Geometry check sheet. Reference: the model listing, model coordinates, mm. Round coordinates to 2 decimals unless told otherwise and drop trailing zeros. One line per question, with ' | ' between items.
```python
from build123d import *

# Parameters (mm, degrees)
LOFT_START          = -150
LOFT_18_DEPTH       = 150
FILLET_1_R          = 50
SKETCH_8_W          = 150
SKETCH_8_H          = 89.90044461
CUT_EXTRUDE_3_DEPTH = 194.637322649
FILLET_3_R          = 10
EXTRUDE_1_REACH     = 195.637
SKETCH_5_R          = 5


# Read off the part's stored shape, not the designer's step: 放样18
with BuildPart() as part:
    # 放样18 outline → 放样18 (new body)
    with BuildSketch(Plane.YZ.offset(LOFT_START)):
        with BuildLine():
            Line((-92.019059125, 77.475043518), (-94.7292742, 73.273289807))
            add(Edge.make_bspline(
                [(-2.5, 0), (-30.482362978, 27.663701514), (-61.402130233, 52.230749004), (-94.7292742, 73.273289807)],
                knots=[0, 0, 0, 0, 1, 1, 1, 1], degree=3))
            Line((-2.5, 0), (2.5, 0))
            add(Edge.make_bspline(
                [(2.5, 0), (-26.24562462, 29.064286084), (-57.928653516, 55.031918144), (-92.019059125, 77.475043518)],
                knots=[0, 0, 0, 0, 1, 1, 1, 1], degree=3))
        make_face()
    extrude(amount=LOFT_18_DEPTH)

    # 圆角1
    fillet_1_edges = [part.edges().sort_by_distance(p)[0] for p in [
        (-150, -93.374166663, 75.374166663),
    ]]
    fillet(fillet_1_edges, radius=FILLET_1_R)

    # 草图8 → 切除-拉伸3 (cut, through all)
    with BuildSketch(Plane(origin=(0, -17.799060008, -17.799060008), x_dir=(-1, 0, 0), z_dir=(0, 0.7071067811865488, 0.7071067811865464))):
        with Locations((75, -43.182455352)):
            Rectangle(SKETCH_8_W, SKETCH_8_H)
    extrude(amount=CUT_EXTRUDE_3_DEPTH, mode=Mode.SUBTRACT)

    # 圆角3
    fillet_3_edges = [part.edges().sort_by_distance(p)[0] for p in [
        (0, -93.374166663, 75.374166663),
        (0, -1.246870677, 1.253129323),
        (-150, -1.246870677, 1.253129323),
    ]]
    fillet(fillet_3_edges, radius=FILLET_3_R)

    # 草图5 → 凸台-拉伸1 (add, up to next)
    with BuildSketch(Plane(origin=(0, -17.799060008, -17.799060008), x_dir=(-1, 0, 0), z_dir=(0, 0.7071067811865488, 0.7071067811865464)), mode=Mode.PRIVATE) as extrude_1_sk1:
        with Locations(Location((140, 11.767766953, 0), (0, 0, 270))):
            Circle(SKETCH_5_R)
    extrude_1_tool1 = extrude(extrude_1_sk1.sketch, amount=EXTRUDE_1_REACH, mode=Mode.PRIVATE) - part.part
    # 草图5 → 凸台-拉伸1 (add, up to next)
    with BuildSketch(Plane(origin=(0, -17.799060008, -17.799060008), x_dir=(-1, 0, 0), z_dir=(0, 0.7071067811865488, 0.7071067811865464)), mode=Mode.PRIVATE) as extrude_1_sk2:
        with Locations(Location((10, 11.767766953, 0), (0, 0, 270))):
            Circle(SKETCH_5_R)
    extrude_1_tool2 = extrude(extrude_1_sk2.sketch, amount=EXTRUDE_1_REACH, mode=Mode.PRIVATE) - part.part
    # 草图5 → 凸台-拉伸1 (add, up to next)
    with BuildSketch(Plane(origin=(0, -17.799060008, -17.799060008), x_dir=(-1, 0, 0), z_dir=(0, 0.7071067811865488, 0.7071067811865464)), mode=Mode.PRIVATE) as extrude_1_sk3:
        with Locations(Location((10, 110.037688609, 0), (0, 0, 270))):
            Circle(SKETCH_5_R)
    extrude_1_tool3 = extrude(extrude_1_sk3.sketch, amount=EXTRUDE_1_REACH, mode=Mode.PRIVATE) - part.part
    # 草图5 → 凸台-拉伸1 (add, up to next)
    with BuildSketch(Plane(origin=(0, -17.799060008, -17.799060008), x_dir=(-1, 0, 0), z_dir=(0, 0.7071067811865488, 0.7071067811865464)), mode=Mode.PRIVATE) as extrude_1_sk4:
        with Locations(Location((100, 70.425532461, 0), (0, 0, 270))):
            Circle(SKETCH_5_R)
    extrude_1_tool4 = extrude(extrude_1_sk4.sketch, amount=EXTRUDE_1_REACH, mode=Mode.PRIVATE) - part.part
    add(extrude_1_tool1.solids().sort_by_distance((-140, -26.120128, -9.477992))[0])
    add(extrude_1_tool2.solids().sort_by_distance((-10, -26.120128, -9.477992))[0])
    add(extrude_1_tool3.solids().sort_by_distance((-10, -95.607456, 60.009336))[0])
    add(extrude_1_tool4.solids().sort_by_distance((-100, -67.597432, 31.999312))[0])


solid = part.part
```
(1) Sectioned sample at A-A on y = -14.5. Count the separate pieces of the cut face and the enclosed holes in it, then the cut area to 3 significant figures.
Resolved:
separate pieces: 3 | enclosed holes: 0 | area: 973 mm2
(2) Draft check along X on faces 1 (the flat face through (-140.1, -26.2, -9.4)), 2 (the cylindrical face through (-134.964, -81.498, 67.481)), 3 (the cylindrical face through (-13.379, -20.585, 1.269)). Enter one of: +X half, -X half, draft (parallel to the pull), parting line (faces both ways), or undercut.
Resolved:
face 1: draft | face 2: -X half | face 3: undercut
(3) Material ranges on line 1 (Z direction, x = -38.5, y = -15); line 2 (Y direction, x = -69.5, z = 42); line 3 (Y direction, x = -61.5, z = 37.5), recorded low to high.
Resolved:
line 1: z = 11.97 to 16.97 | line 2: y = -50.27 to -43.71 | line 3: y = -44.58 to -38.26
(4) Go/stop test with flat-tipped pins: pin 1 (1.5 mm diameter, centred on x = -43, y = -26.5, fed in from -Z); pin 2 (3 mm diameter, centred on x = -117.5, y = -76.5, fed in from +Z); pin 3 (4 mm diameter, centred on x = -116.5, z = 49, fed in from -Y); pin 4 (6 mm diameter, centred on y = -49.5, z = 34.5, fed in from +X). Record where each tip stops, or that it passes through.
Resolved:
pin 1: stops at z = 21.68 | pin 2: stops at z = 67.95 | pin 3: stops at y = -62.13 | pin 4: passes through
